Autodesk Inventor part; units mm, degrees
ref_plane "YZ Plane" through (0, 0, 0) normal (1, 0, 0) x (0, 1, 0)
ref_plane "XZ Plane" through (0, 0, 0) normal (0, 1, 0) x (-1, 0, 0)
ref_plane "XY Plane" through (0, 0, 0) normal (0, 0, 1) x (1, 0, 0)
sketch "Sketch1" plane through (0, 0, 0) normal (0, 0, 1) x (1, 0, 0)
  line L0 (-6.35, -6.35) -> (6.35, -6.35)
  line L1 (6.35, -6.35) -> (6.35, 6.35)
  line L2 (6.35, 6.35) -> (-6.35, 6.35)
  line L3 (-6.35, 6.35) -> (-6.35, -6.35)
  line L4 (-6.35, -6.35) -> (6.35, 6.35) construction
  line L5 (6.35, -6.35) -> (-6.35, 6.35) construction
  line L6 (-0.3534, 2.4749) -> (-0.4996, 2.1425)
  line L7 (-0.3534, 2.4749) -> (-0.12, 2.1967)
  line L8 (-0.7778, 2.3759) -> (-0.8641, 2.0232)
  line L9 (-0.7778, 2.3759) -> (-0.4996, 2.1425)
  line L10 (-1.1786, 2.2048) -> (-1.2023, 1.8424)
  line L11 (-1.1786, 2.2048) -> (-0.8641, 2.0232)
  line L12 (-1.5435, 1.9666) -> (-1.504, 1.6056)
  line L13 (-1.5435, 1.9666) -> (-1.2023, 1.8424)
  line L14 (-1.8616, 1.6687) -> (-1.7599, 1.3201)
  line L15 (-1.8616, 1.6687) -> (-1.504, 1.6056)
  line L16 (-2.1231, 1.3201) -> (-1.9624, 0.9944)
  line L17 (-2.1231, 1.3201) -> (-1.7599, 1.3201)
  line L18 (-2.32, 0.9314) -> (-2.1053, 0.6386)
  line L19 (-2.32, 0.9314) -> (-1.9624, 0.9944)
  line L20 (-2.4465, 0.5144) -> (-2.1842, 0.2633)
  line L21 (-2.4465, 0.5144) -> (-2.1053, 0.6386)
  line L22 (-2.4987, 0.0817) -> (-2.1967, -0.12)
  line L23 (-2.4987, 0.0817) -> (-2.1842, 0.2633)
  line L24 (-2.4749, -0.3534) -> (-2.1425, -0.4996)
  line L25 (-2.4749, -0.3534) -> (-2.1967, -0.12)
  line L26 (-2.3759, -0.7778) -> (-2.0232, -0.8641)
  line L27 (-2.3759, -0.7778) -> (-2.1425, -0.4996)
  line L28 (-2.2048, -1.1786) -> (-1.8424, -1.2023)
  line L29 (-2.2048, -1.1786) -> (-2.0232, -0.8641)
  line L30 (-1.9666, -1.5435) -> (-1.6056, -1.504)
  line L31 (-1.9666, -1.5435) -> (-1.8424, -1.2023)
  line L32 (-1.6687, -1.8616) -> (-1.3201, -1.7599)
  line L33 (-1.6687, -1.8616) -> (-1.6056, -1.504)
  line L34 (-1.3201, -2.1231) -> (-0.9944, -1.9624)
  line L35 (-1.3201, -2.1231) -> (-1.3201, -1.7599)
  line L36 (-0.9314, -2.32) -> (-0.6386, -2.1053)
  line L37 (-0.9314, -2.32) -> (-0.9944, -1.9624)
  line L38 (-0.5144, -2.4465) -> (-0.2633, -2.1842)
  line L39 (-0.5144, -2.4465) -> (-0.6386, -2.1053)
  line L40 (-0.0817, -2.4987) -> (0.12, -2.1967)
  line L41 (-0.0817, -2.4987) -> (-0.2633, -2.1842)
  line L42 (0.3534, -2.4749) -> (0.4996, -2.1425)
  line L43 (0.3534, -2.4749) -> (0.12, -2.1967)
  line L44 (0.7778, -2.3759) -> (0.8641, -2.0232)
  line L45 (0.7778, -2.3759) -> (0.4996, -2.1425)
  line L46 (1.1786, -2.2048) -> (1.2023, -1.8424)
  line L47 (1.1786, -2.2048) -> (0.8641, -2.0232)
  line L48 (1.5435, -1.9666) -> (1.504, -1.6056)
  line L49 (1.5435, -1.9666) -> (1.2023, -1.8424)
  line L50 (1.8616, -1.6687) -> (1.7599, -1.3201)
  line L51 (1.8616, -1.6687) -> (1.504, -1.6056)
  line L52 (2.1231, -1.3201) -> (1.9624, -0.9944)
  line L53 (2.1231, -1.3201) -> (1.7599, -1.3201)
  line L54 (2.32, -0.9314) -> (2.1053, -0.6386)
  line L55 (2.32, -0.9314) -> (1.9624, -0.9944)
  line L56 (2.4465, -0.5144) -> (2.1842, -0.2633)
  line L57 (2.4465, -0.5144) -> (2.1053, -0.6386)
  line L58 (2.4987, -0.0817) -> (2.1967, 0.12)
  line L59 (2.4987, -0.0817) -> (2.1842, -0.2633)
  line L60 (2.4749, 0.3534) -> (2.1425, 0.4996)
  line L61 (2.4749, 0.3534) -> (2.1967, 0.12)
  line L62 (2.3759, 0.7778) -> (2.0232, 0.8641)
  line L63 (2.3759, 0.7778) -> (2.1425, 0.4996)
  line L64 (2.2048, 1.1786) -> (1.8424, 1.2023)
  line L65 (2.2048, 1.1786) -> (2.0232, 0.8641)
  line L66 (1.9666, 1.5435) -> (1.6056, 1.504)
  line L67 (1.9666, 1.5435) -> (1.8424, 1.2023)
  line L68 (1.6687, 1.8616) -> (1.3201, 1.7599)
  line L69 (1.6687, 1.8616) -> (1.6056, 1.504)
  line L70 (1.3201, 2.1231) -> (0.9944, 1.9624)
  line L71 (1.3201, 2.1231) -> (1.3201, 1.7599)
  line L72 (0.9314, 2.32) -> (0.6386, 2.1053)
  line L73 (0.9314, 2.32) -> (0.9944, 1.9624)
  line L74 (0.5144, 2.4465) -> (0.2633, 2.1842)
  line L75 (0.5144, 2.4465) -> (0.6386, 2.1053)
  line L76 (0.0817, 2.4987) -> (-0.12, 2.1967)
  line L77 (0.0817, 2.4987) -> (0.2633, 2.1842)
  circle A0 centre (0, 0) radius 0.3723
  point P0 (0, 0)
  dimension "d0" = 12.7
  dimension "d1" = 12.7
extrude "Extrusion1" add sketch "Sketch1" along normal blind 3.5 contours L3 L2 L1 L0 | L7 L76 L77 L74 L75 L72 L73 L70 L71 L68 L69 L66 L67 L64 L65 L62 L63 L60 L61 L58 L59 L56 L57 L54 L55 L52 L53 L50 L51 L48 L49 L46 L47 L44 L45 L42 L43 L40 L41 L38 L39 L36 L37 L34 L35 L32 L33 L30 L31 L28 L29 L26 L27 L24 L25 L22 L23 L20 L21 L18 L19 L16 L17 L14 L15 L12 L13 L10 L11 L8 L9 L6 | A0
sketch "Sketch2" plane through (0, 0, 3.5) normal (0, 0, 1) x (1, 0, 0)
  line L0 (2.2048, 1.1786) -> (1.8424, 1.2023)
  line L1 (2.2048, 1.1786) -> (2.0232, 0.8641)
  line L2 (2.4749, 0.3534) -> (2.1425, 0.4996)
  line L3 (2.4749, 0.3534) -> (2.1967, 0.12)
  line L4 (2.4987, -0.0817) -> (2.1967, 0.12)
  line L5 (2.4987, -0.0817) -> (2.1842, -0.2633)
  line L6 (-0.3534, 2.4749) -> (-0.12, 2.1967)
  line L7 (-0.3534, 2.4749) -> (-0.4996, 2.1425)
  line L8 (-1.5435, 1.9666) -> (-1.504, 1.6056)
  line L9 (-1.8616, 1.6687) -> (-1.504, 1.6056)
  line L10 (-1.8616, 1.6687) -> (-1.7599, 1.3201)
  line L11 (-1.5435, 1.9666) -> (-1.2023, 1.8424)
  line L12 (-1.1786, 2.2048) -> (-1.2023, 1.8424)
  line L13 (-1.1786, 2.2048) -> (-0.8641, 2.0232)
  line L14 (-0.7778, 2.3759) -> (-0.8641, 2.0232)
  line L15 (-0.7778, 2.3759) -> (-0.4996, 2.1425)
  line L16 (-2.1231, 1.3201) -> (-1.7599, 1.3201)
  line L17 (-2.1231, 1.3201) -> (-1.9624, 0.9944)
  line L18 (-2.32, 0.9314) -> (-1.9624, 0.9944)
  line L19 (-2.32, 0.9314) -> (-2.1053, 0.6386)
  line L20 (-2.4465, 0.5144) -> (-2.1053, 0.6386)
  line L21 (-2.4465, 0.5144) -> (-2.1842, 0.2633)
  line L22 (-2.4987, 0.0817) -> (-2.1842, 0.2633)
  line L23 (-2.4987, 0.0817) -> (-2.1967, -0.12)
  line L24 (-2.4749, -0.3534) -> (-2.1967, -0.12)
  line L25 (-2.4749, -0.3534) -> (-2.1425, -0.4996)
  line L26 (-2.3759, -0.7778) -> (-2.1425, -0.4996)
  line L27 (-2.3759, -0.7778) -> (-2.0232, -0.8641)
  line L28 (-2.2048, -1.1786) -> (-2.0232, -0.8641)
  line L29 (-2.2048, -1.1786) -> (-1.8424, -1.2023)
  line L30 (-1.9666, -1.5435) -> (-1.8424, -1.2023)
  line L31 (-1.9666, -1.5435) -> (-1.6056, -1.504)
  line L32 (-1.6687, -1.8616) -> (-1.6056, -1.504)
  line L33 (-1.6687, -1.8616) -> (-1.3201, -1.7599)
  line L34 (-1.3201, -2.1231) -> (-1.3201, -1.7599)
  line L35 (-1.3201, -2.1231) -> (-0.9944, -1.9624)
  line L36 (-0.9314, -2.32) -> (-0.9944, -1.9624)
  line L37 (-0.9314, -2.32) -> (-0.6386, -2.1053)
  line L38 (-0.5144, -2.4465) -> (-0.6386, -2.1053)
  line L39 (-0.5144, -2.4465) -> (-0.2633, -2.1842)
  line L40 (-0.0817, -2.4987) -> (-0.2633, -2.1842)
  line L41 (-0.0817, -2.4987) -> (0.12, -2.1967)
  line L42 (0.3534, -2.4749) -> (0.12, -2.1967)
  line L43 (0.3534, -2.4749) -> (0.4996, -2.1425)
  line L44 (0.7778, -2.3759) -> (0.4996, -2.1425)
  line L45 (0.7778, -2.3759) -> (0.8641, -2.0232)
  line L46 (1.1786, -2.2048) -> (0.8641, -2.0232)
  line L47 (1.1786, -2.2048) -> (1.2023, -1.8424)
  line L48 (1.5435, -1.9666) -> (1.2023, -1.8424)
  line L49 (1.5435, -1.9666) -> (1.504, -1.6056)
  line L50 (1.8616, -1.6687) -> (1.504, -1.6056)
  line L51 (1.8616, -1.6687) -> (1.7599, -1.3201)
  line L52 (2.1231, -1.3201) -> (1.7599, -1.3201)
  line L53 (2.1231, -1.3201) -> (1.9624, -0.9944)
  line L54 (2.32, -0.9314) -> (1.9624, -0.9944)
  line L55 (2.32, -0.9314) -> (2.1053, -0.6386)
  line L56 (2.4465, -0.5144) -> (2.1053, -0.6386)
  line L57 (2.4465, -0.5144) -> (2.1842, -0.2633)
  line L58 (2.3759, 0.7778) -> (2.0232, 0.8641)
  line L59 (2.3759, 0.7778) -> (2.1425, 0.4996)
  line L60 (1.9666, 1.5435) -> (1.8424, 1.2023)
  line L61 (1.9666, 1.5435) -> (1.6056, 1.504)
  line L62 (1.6687, 1.8616) -> (1.6056, 1.504)
  line L63 (1.6687, 1.8616) -> (1.3201, 1.7599)
  line L64 (0.0817, 2.4987) -> (-0.12, 2.1967)
  line L65 (0.0817, 2.4987) -> (0.2633, 2.1842)
  circle A0 centre (0, 0) radius 0.3723
  line L66 (0.5144, 2.4465) -> (0.2633, 2.1842)
  line L67 (0.5144, 2.4465) -> (0.6386, 2.1053)
  line L68 (1.3201, 2.1231) -> (1.3201, 1.7599)
  line L69 (1.3201, 2.1231) -> (0.9944, 1.9624)
  line L70 (0.9314, 2.32) -> (0.9944, 1.9624)
  line L71 (0.9314, 2.32) -> (0.6386, 2.1053)
  point P0 (0, 0)
extrude "Extrusion2" cut sketch "Sketch2" against normal blind 3.2 contours L1 L58 L59 L2 L3 L4 L5 L57 L56 L55 L54 L53 L52 L51 L50 L49 L48 L47 L46 L45 L44 L43 L42 L41 L40 L39 L38 L37 L36 L35 L34 L33 L32 L31 L30 L29 L28 L27 L26 L25 L24 L23 L22 L21 L20 L19 L18 L17 L16 L10 L9 L8 L11 L12 L13 L14 L15 L7 L6 L64 L65 L66 L67 L71 L70 L69 L68 L63 L62 L61 L60 L0 | A0
chamfer "Chamfer1" distance 3.175 angle 45 4 edges at (0, -6.35, 3.5) (-6.35, 0, 3.5) (6.35, 0, 3.5) (0, 6.35, 3.5)
properties part number "Servo Grip"
Geometry check sheet. Reference: the model listing, model coordinates, mm. Round coordinates to 2 decimals unless told otherwise and drop trailing zeros. Loops run counter-clockwise (first coordinate to the right, second up) from the corner with the lowest first, then second, coordinate; pieces in that order, holes last. Notation, with made-up numbers: M 65,-23 L 110,-23 A23 ccw 110,-3 Z; hole C 77,-16.5 d6. An arc over 180 degrees is marked long. Return JSON: item names as keys, results as strings. Group by question number.
(1) Go/stop test with flat-tipped pins: pin 1 (1.5 mm diameter, centred on y = -1.5, z = 3, fed in from +X) (3 decimals); pin 2 (2 mm diameter, centred on y = -1.5, z = 2, fed in from -X) (3 decimals); pin 3 (1.5 mm diameter, centred on x = -1, y = 1, fed in from +Z). Record where each tip stops, or that it passes through.
(2) Mould release check, pull along X, two halves, no side actions. Record for faces 1 (the face through (0, 0, 0.3)), 2 (the face through (-1.5, 2.2, 3.5)), 3 (the face through (5.138, -0.089, 1.537)): pulls with the +X half, pulls with the -X half, needs draft (parallel to the pull), parting line crosses it, or undercut.
(3) Section check A-A, the plane x = -3.5. Enter the section's corners in (y, z) (3 decimals), and give its area (3 significant figures).
(4) Scan lines: line 1 along Z through (x, y) = (3, -3.5) (3 decimals); line 2 along X through (y, z) = (0.75, 3.1) (3 decimals); line 3 along Y through (x, z) = (0.75, 1.85) (3 decimals). Record each from-to range of solid material in increasing order. Write a range as [from, to].
Data:
{
 "1": {"pin 1": "x = 4.425", "pin 2": "x = -5.675", "pin 3": "z = 0.3"},
 "2": {"face 1": "undercut", "face 2": "needs draft", "face 3": "pulls with the +X half"},
 "3": {"outline": "M -6.35,0 L 6.35,0 L 6.35,0.325 L 3.5,3.175 L -3.5,3.175 L -6.35,0.325 Z", "area": "32.2 mm²"},
 "4": {"line 1": "[0, 3.175]", "line 2": "[-3.575, -2.187], [2.353, 3.575]", "line 3": "[-4.825, -2.353], [2.187, 4.825]"}
}
